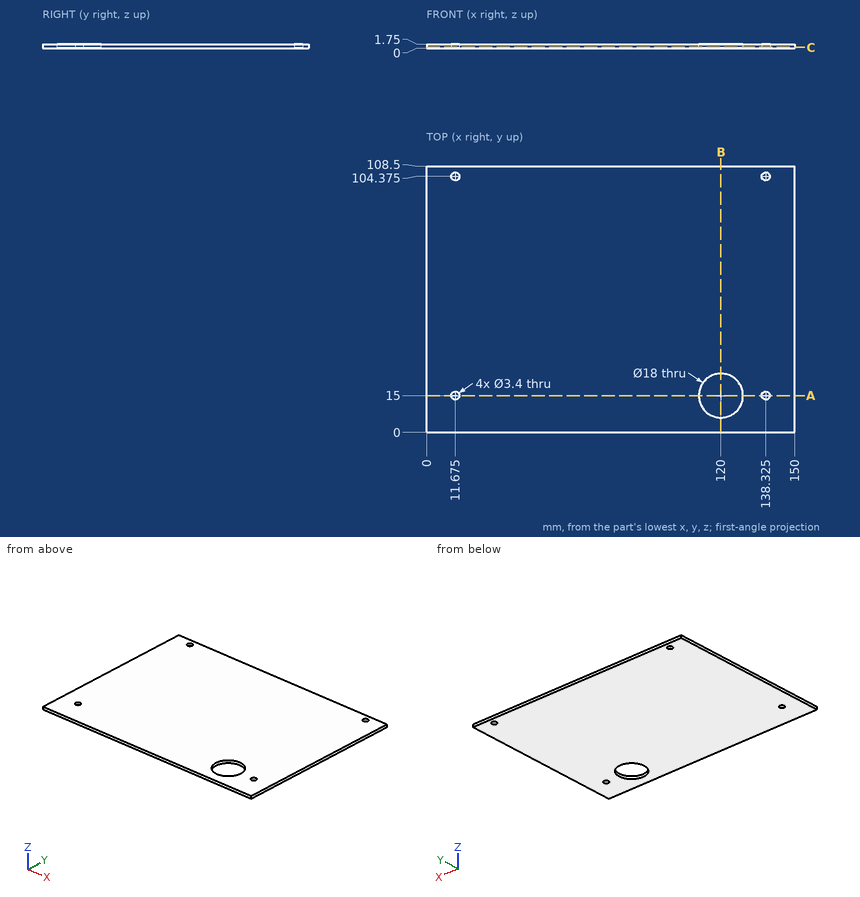
Print and shaded views of the part. All mm, measured from the part's lowest x, y and z. Round coordinates to 2 decimals unless told otherwise and drop trailing zeros. Write each loop counter-clockwise with the first axis right and the second up, starting at its lowest first coordinate (ties: lowest second). Pieces come first, ordered by that corner, then holes. Notation, with made-up numbers: (45.5, -4.75) - (75.5, -4.75) arc R30 ccw to (75.5, 24.25) - close; hole circle Ø3 at (-23, 50.25). An arc over 180 degrees is marked (long way). One line per question, with ' | ' between items.
1. Band-saw the part on C-C, the plane z = 0.35. Write the cut outline in (x, y) (3 decimals), and give its area (3 significant figures).
Results are:
outline: (0, 0) - (150, 0) - (150, 108.5) - (0, 108.5) - close; hole circle Ø3.4 at (11.675, 15); hole circle Ø3.4 at (11.675, 104.375); hole circle Ø18 at (120, 15); hole circle Ø3.4 at (138.325, 15); hole circle Ø3.4 at (138.325, 104.375) | area: 16,000 mm^2
2. Band-saw the part on A-A, the plane y = 15. Write the cut outline in (x, z) (3 decimals), and give its area (3 significant figures).
Results are:
outline: (0, 0) - (9.975, 0) - (9.975, 1.75) - (0, 1.75) - close; (13.375, 0) - (111, 0) - (111, 1.75) - (13.375, 1.75) - close; (129, 0) - (136.625, 0) - (136.625, 1.75) - (129, 1.75) - close; (140.025, 0) - (150, 0) - (150, 1.75) - (140.025, 1.75) - close | area: 219 mm^2
3. Drill centre lines: line 1 along Y through (x, z) = (120, 1.1); line 2 along X through (y, z) = (14, 1); line 3 along Y through (x, z) = (128, 0.5). Where is each one in solid material? Low to high. Write a range as from..to.
Results are:
line 1: 0..6, 24..108.5 | line 2: 0..10.3, 13.05..111.06, 128.94..136.95, 139.7..150 | line 3: 0..10.88, 19.12..108.5
4. Drop a flat-ended pin along its axis: pin 1 Ø2 at (x, y) = (138.325, 15) entering from +Z. Give the stop position or say it passes through.
Results are:
pin 1: through
5. Band-saw the part on B-B, the plane x = 120. Write the cut outline in (y, z), and give its area (3 significant figures).
Results are:
outline: (0, 0) - (6, 0) - (6, 1.75) - (0, 1.75) - close; (24, 0) - (108.5, 0) - (108.5, 1.75) - (24, 1.75) - close | area: 158 mm^2
